```python
from build123d import *

# Parameters (mm, degrees)
SKETCH2_R           = 9.75
SKETCH2_R_2         = 4
BOSS_EXTRUDE1_DEPTH = 3
SKETCH3_R           = 5.5
SKETCH3_R_2         = 3
BOSS_EXTRUDE2_DEPTH = 10
SKETCH16_R          = 9.75
SKETCH16_R_2        = 5.5
BOSS_EXTRUDE3_DEPTH = 2
SKETCH5_R           = 1.1
CUT_EXTRUDE1_DEPTH  = 16.941298617


# Read off the part's stored shape, not the designer's step: M3x0.5 Tapped Hole1
with BuildPart() as part:
    # Sketch2 → Boss-Extrude1 (new body)
    with BuildSketch(Plane(origin=(0, 0, 0), x_dir=(1, 0, 0), z_dir=(0, 1, 0))):
        with Locations(Location((0, 0, 0), (0, 0, 270))):
            Circle(SKETCH2_R)
        with Locations(Location((0, 0, 0), (0, 0, 270))):
            Circle(SKETCH2_R_2, mode=Mode.SUBTRACT)
    extrude(amount=BOSS_EXTRUDE1_DEPTH)

    # Sketch3 → Boss-Extrude2 (add)
    with BuildSketch(Plane(origin=(0, 3, 0), x_dir=(1, 0, 0), z_dir=(0, 1, 0))):
        with Locations(Location((0, 0, 0), (0, 0, 270))):
            Circle(SKETCH3_R)
        with Locations(Location((0, 0, 0), (0, 0, 270))):
            Circle(SKETCH3_R_2, mode=Mode.SUBTRACT)
    extrude(amount=BOSS_EXTRUDE2_DEPTH)

    # Sketch16 → Boss-Extrude3 (add)
    with BuildSketch(Plane(origin=(0, 3, 0), x_dir=(1, 0, 0), z_dir=(0, 1, 0))):
        with Locations(Location((0, 0, 0), (0, 0, 270))):
            Circle(SKETCH16_R)
        with Locations(Location((0, 0, 0), (0, 0, 270))):
            Circle(SKETCH16_R_2, mode=Mode.SUBTRACT)
    extrude(amount=BOSS_EXTRUDE3_DEPTH)

    # M3x0.5 Tapped Hole1 outline → M3x0.5 Tapped Hole1 (revolve, cut)
    with BuildSketch(Plane.XZ.offset(-9)):
        Polygon((1.525000456, 5.500000456), (0, 5.500000456), (0, 2.727054604), (1.25, 2.727054604), (1.25, 5.225), align=None)
    revolve(axis=Axis((0, 9, 0), (0, 0, 1)), mode=Mode.SUBTRACT)

    # Sketch5 → Cut-Extrude1 (cut, through all)
    with BuildSketch(Plane(origin=(0, 5, 0), x_dir=(1, 0, 0), z_dir=(0, 1, 0))):
        with Locations(Location((3.061467459, 7.39103626, 0), (0, 0, 270))):
            Circle(SKETCH5_R)
        with Locations(Location((7.39103626, 3.061467459, 0), (0, 0, 270))):
            Circle(SKETCH5_R)
        with Locations(Location((7.39103626, -3.061467459, 0), (0, 0, 270))):
            Circle(SKETCH5_R)
        with Locations(Location((3.061467459, -7.39103626, 0), (0, 0, 270))):
            Circle(SKETCH5_R)
        with Locations(Location((-3.061467459, -7.39103626, 0), (0, 0, 270))):
            Circle(SKETCH5_R)
        with Locations(Location((-7.39103626, -3.061467459, 0), (0, 0, 270))):
            Circle(SKETCH5_R)
        with Locations(Location((-7.39103626, 3.061467459, 0), (0, 0, 270))):
            Circle(SKETCH5_R)
        with Locations(Location((-3.061467459, 7.39103626, 0), (0, 0, 270))):
            Circle(SKETCH5_R)
    extrude(amount=-CUT_EXTRUDE1_DEPTH, mode=Mode.SUBTRACT)


solid = part.part
```
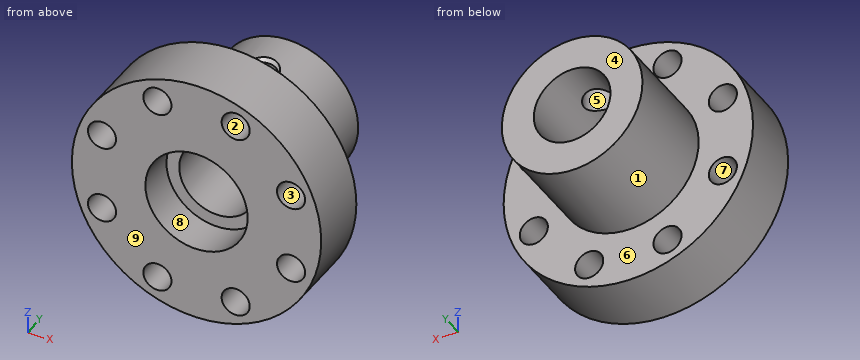
Input: part model. Units: mm. Frame: model coordinates. Face numbers are marked on the shaded views. A direction names the side the tool comes from. Give positions to 0.01 mm unless a question says otherwise; leave off trailing zeros. Order: outer loops, then holes, each group sorted by start corner. A loop starts at its lowest first (then second) coordinate and runs counter-clockwise, first axis right, second up.
1. Set-up query: the marked faces 5, 6, 7, 8 and 9. Return all of +Z, -Z, +X, -X, +Y, -Y with unobstructed straight access to the full face (end or side cutting, diameter ignored); none if empty.
Computed:
face 5: +Z
face 6: +Y
face 7: +Y, -Y
face 8: -Y
face 9: +Z, -Z, +X, -X, -Y
2. Cut plane A-A (x = 0). Return loops of the section in (y, z) (3 decimals).
Computed:
outline: (0, -9.75) - (5, -9.75) - (5, -5.5) - (13, -5.5) - (13, -3) - (3, -3) - (3, -4) - (0, -4) - close; (0, 4) - (3, 4) - (3, 3) - (7.75, 3) - (7.75, 5.225) - (7.475, 5.5) - (5, 5.5) - (5, 9.75) - (0, 9.75) - close; (10.25, 3) - (13, 3) - (13, 5.5) - (10.525, 5.5) - (10.25, 5.225) - close
3. Draft query along X for the marked faces 1, 2, 3 and 4. Return one class per face: released by +X, released by -X, zero draft, split by the parting line, or undercut.
Computed:
face 1: split by the parting line
face 2: undercut
face 3: undercut
face 4: zero draft
4. Pin query (flat end, axial travel): pin 1 Ø1 at (x, y) = (-3, 9) entering from +Z; pin 2 Ø1 at (x, y) = (-3.5, 10) entering from +Z; pin 3 Ø1.5 at (x, z) = (-4, 7.5) entering from +Y. Return the tip coordinate at first contact, or that it passes through.
Computed:
pin 1: stops at z = 4.9
pin 2: stops at z = 4.61
pin 3: stops at y = 5
5. Cut plane B-B (z = 0). Return loops of the section in (x, y).
Computed:
outline: (-9.75, 0) - (-4, 0) - (-4, 3) - (-3, 3) - (-3, 13) - (-5.5, 13) - (-5.5, 5) - (-9.75, 5) - close; (3, 3) - (4, 3) - (4, 0) - (9.75, 0) - (9.75, 5) - (5.5, 5) - (5.5, 13) - (3, 13) - close
6. Cut plane D-D (y = 1.75). State how many separate pieces and enclosed holes the cut face has, and give its area (3 significant figures).
Computed:
separate pieces: 1
enclosed holes: 9
area: 218 mm2
7. Line query: probe 1 along X at (y, z) = (6.5, 0); probe 2 along Y at (x, z) = (7.5, 5); probe 3 along Z at (x, y) = (-6.75, 3.5). Output: solid intervals per line, ascending.
Computed:
probe 1: x = -5.5 to -3, 3 to 5.5
probe 2: y = 0 to 5
probe 3: z = -7.04 to -3.96, -2.17 to 2.17, 3.96 to 7.04
8. Cut plane C-C (z = -7.5). Return loops of the section in (x, y).
Computed:
outline: (-6.23, 0) - (-4.16, 0) - (-4.16, 5) - (-6.23, 5) - close; (-1.97, 0) - (1.97, 0) - (1.97, 5) - (-1.97, 5) - close; (4.16, 0) - (6.23, 0) - (6.23, 5) - (4.16, 5) - close
